The listing builds one solid part. Answer for the finished solid, in the listing's coordinates (mm). Face numbers are marked on the shaded views. Round coordinates to 2 decimals unless told otherwise and drop trailing zeros. Loops run counter-clockwise (first coordinate to the right, second up) from the corner with the lowest first, then second, coordinate; pieces in that order, holes last. Notation, with made-up numbers: M 6,-23 L 22,-23 A22 ccw 22,-16 Z; hole C 37.25,21.5 d8. An arc over 180 degrees is marked long. Answer as a JSON object with one key per item and string values.
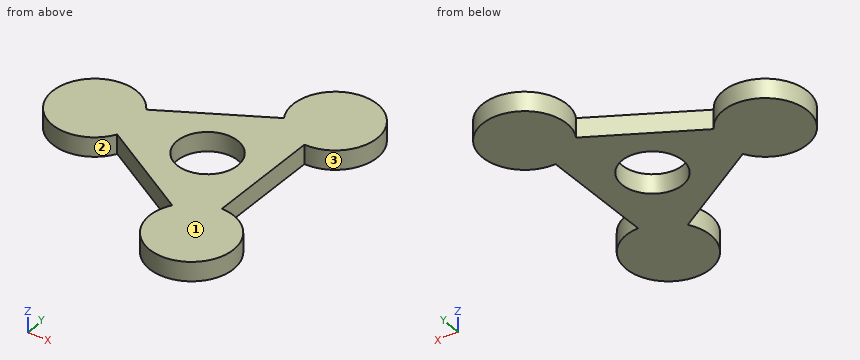
```python
from build123d import *

# Parameters (mm, degrees)
F1_DEPTH = 7.0104
F2_D     = 22.06
F3_R     = 15.305
F4_DEPTH = 7.0104


with BuildPart() as f1:
    # F0 (on Top) → F1 (new body)
    with BuildSketch(Plane.XY):
        Polygon((21.226586, 35.185908), (-41.085183, 0.789809), (19.858597, -35.975717), align=None)
    extrude(amount=F1_DEPTH)

    # F2 (through all)
    with Locations(Plane(origin=(0, 0, 0), x_dir=(1, 0, 0), z_dir=(0, 0, -1))):
        with Locations((0, 0)):
            Hole(F2_D / 2)

    # F3 (on Top) → F4 (join)
    with BuildSketch(Plane.XY):
        with Locations((21.35277, 35.396876)):
            Circle(F3_R)
        with Locations((-40.842548, 0)):
            Circle(F3_R)
        with Locations((19.9197, -36.543333)):
            Circle(F3_R)
    extrude(amount=F4_DEPTH)


solid = f1.part
```
Item 1: Determine the mould class of the marked faces 1, 2 and 3 for opening direction X: released by +X, released by -X, zero draft, split by the parting line, or undercut.
Values follow:
{"face 1": "zero draft", "face 2": "undercut", "face 3": "split by the parting line"}
Item 2: The part is cut by section A-A (y = 14). Give the vertices of the cut face in (x, z).
Values follow:
{"outline": "M -47.03,0 L -34.66,0 L -34.66,7.01 L -47.03,7.01 Z; M -17.15,0 L 20.82,0 L 20.82,7.01 L -17.15,7.01 Z"}
Item 3: The part is cut by section C-C (z = 5.5). Give the vertices of the cut face in (x, y) (3 decimals).
Values follow:
{"outline": "M -27.853,8.094 A15.305 ccw long -27.461,-7.429 L 7.055,-28.252 A15.305 ccw long 20.142,-21.24 L 20.937,20.098 A15.305 ccw long 8.014,27.892 Z; hole C 0,0 d22.06"}
Item 4: The part is cut by section D-D (y = -26). Give the vertices of the cut face in (x, z).
Values follow:
{"outline": "M 3.32,0 L 31.01,0 L 31.01,7.01 L 3.32,7.01 Z"}
Item 5: The part is cut by section B-B (x = 0). Give the vertices of the cut face in (y, z), then the cut area to 3 significant figures.
Values follow:
{"outline": "M -24,0 L -11.03,0 L -11.03,7.01 L -24,7.01 Z; M 11.03,0 L 23.47,0 L 23.47,7.01 L 11.03,7.01 Z", "area": "178 mm^2"}
Item 6: Straight lines are drawn through the part: line 1 (X direction, y = 10, z = 2.5); line 2 (X direction, y = -8.5, z = 5.5); line 3 (X direction, y = -3.5, z = 6.5). For each, find the intervals that lie inside material, in ascending order.
Values follow:
{"line 1": "-52.43 to -29.26, -24.4 to -4.65, 4.65 to 20.74", "line 2": "-53.57 to -28.11, -25.69 to -7.03, 7.03 to 20.39", "line 3": "-55.74 to -10.46, 10.46 to 20.48"}
Item 7: Flat-ended cylindrical pins translate along their axes: P1, Ø17.5, axis at x = 0, y = 0, coming from the +Z side; P2, Ø3, axis at x = -44, z = 3, coming from the +Y side (3 decimals); P3, Ø1, axis at x = -29, z = 1.5, coming from the +Y side; P4, Ø3, axis at y = 15.5, z = 1.5, coming from the +X side. Find the tip coordinate at first contact, or state that the pin passes through.
Values follow:
{"P1": "through", "P2": "y = 15.215", "P3": "y = 10.28", "P4": "x = 20.88"}
